```python
from build123d import *

# Parameters (mm, degrees)
BOSS_EXTRUDE1_START     = -2.5
SKETCH1_W               = 70
SKETCH1_H               = 39.95
BOSS_EXTRUDE1_DEPTH     = 2.5
SKETCH2_W               = 60
SKETCH2_H               = 2.6
BOSS_EXTRUDE2_DEPTH     = 13.5
SKETCH3_W               = 60
SKETCH3_H               = 2.6
BOSS_EXTRUDE3_DEPTH     = 13.5
SKETCH4_R               = 2.75
BOSS_EXTRUDE4_DEPTH     = 13.5
BOSS_EXTRUDE5_START     = -19
SKETCH5_R               = 5
BOSS_EXTRUDE5_DEPTH     = 16.5
SKETCH6_R               = 3
BOSS_EXTRUDE6_DEPTH     = 22.6
CUT_EXTRUDE1_START      = 14.6
SKETCH7_R               = 0.9
CUT_EXTRUDE1_DEPTH      = 8.1
CUT_EXTRUDE2_DEPTH      = 47.965525921
CUT_EXTRUDE2_DEPTH_BACK = 47.965525921
SKETCH8_W               = 22.8
SKETCH8_H               = 11.9
CUT_EXTRUDE3_DEPTH      = 47.965525921
CUT_EXTRUDE3_DEPTH_BACK = 47.965525921
SKETCH9_R               = 0.9
CUT_EXTRUDE4_DEPTH      = 47.965525921
CUT_EXTRUDE4_DEPTH_BACK = 47.965525921
SKETCH10_R              = 0.9
CUT_EXTRUDE5_DEPTH      = 47.965525921
CUT_EXTRUDE5_DEPTH_BACK = 47.965525921
SKETCH11_R              = 1.725
CUT_EXTRUDE6_START      = -4.2
CUT_EXTRUDE6_DEPTH      = 4.2


with BuildPart() as part:
    # Sketch1 → Boss-Extrude1 (new body)
    with BuildSketch(Plane.XY.offset(BOSS_EXTRUDE1_START)):
        Rectangle(SKETCH1_W, SKETCH1_H)
    extrude(amount=BOSS_EXTRUDE1_DEPTH)

    # Sketch2 → Boss-Extrude2 (add)
    with BuildSketch(Plane.XY):
        with Locations((-5, 16.975)):
            Rectangle(SKETCH2_W, SKETCH2_H)
    extrude(amount=BOSS_EXTRUDE2_DEPTH)

    # Sketch3 → Boss-Extrude3 (add)
    with BuildSketch(Plane.XY):
        with Locations((5, -16.975)):
            Rectangle(SKETCH3_W, SKETCH3_H)
    extrude(amount=BOSS_EXTRUDE3_DEPTH)

    # Sketch4 → Boss-Extrude4 (add)
    with BuildSketch(Plane.XY):
        with Locations((-8, 16.975)):
            Circle(SKETCH4_R)
        with Locations((8, -16.975)):
            Circle(SKETCH4_R)
    extrude(amount=BOSS_EXTRUDE4_DEPTH)

    # Sketch5 → Boss-Extrude5 (add)
    with BuildSketch(Plane.XY.offset(BOSS_EXTRUDE5_START)):
        with Locations(Location((-31, 6, 0), (0, 0, 143.130102354))):
            Circle(SKETCH5_R)
        with Locations(Location((-31, -6, 0), (0, 0, 143.130102354))):
            Circle(SKETCH5_R)
    extrude(amount=BOSS_EXTRUDE5_DEPTH)

    # Sketch6 → Boss-Extrude6 (add)
    with BuildSketch(Plane.XY):
        with Locations((30, 0)):
            Circle(SKETCH6_R)
        with Locations((-30, 0)):
            Circle(SKETCH6_R)
    extrude(amount=BOSS_EXTRUDE6_DEPTH)

    # Sketch7 → Cut-Extrude1 (cut)
    with BuildSketch(Plane.XY.offset(CUT_EXTRUDE1_START)):
        with Locations((30, 0)):
            Circle(SKETCH7_R)
        with Locations((-30, 0)):
            Circle(SKETCH7_R)
    extrude(amount=CUT_EXTRUDE1_DEPTH, mode=Mode.SUBTRACT)

    # Sketch8 → Cut-Extrude2 (cut, two sides: drawn at the far end of the back side and taken through both)
    with BuildSketch(Plane.XY.offset(-CUT_EXTRUDE2_DEPTH_BACK)):
        with Locations((5.8, 0)):
            Rectangle(SKETCH8_W, SKETCH8_H)
    extrude(amount=CUT_EXTRUDE2_DEPTH + CUT_EXTRUDE2_DEPTH_BACK, mode=Mode.SUBTRACT)

    # Sketch9 → Cut-Extrude3 (cut, two sides: drawn at the far end of the back side and taken through both)
    with BuildSketch(Plane.XY.offset(-CUT_EXTRUDE3_DEPTH_BACK)):
        with Locations((-7.95, 0)):
            Circle(SKETCH9_R)
        with Locations((19.55, 0)):
            Circle(SKETCH9_R)
    extrude(amount=CUT_EXTRUDE3_DEPTH + CUT_EXTRUDE3_DEPTH_BACK, mode=Mode.SUBTRACT)

    # Sketch10 → Cut-Extrude4 (cut, two sides: drawn at the far end of the back side and taken through both)
    with BuildSketch(Plane.XY.offset(-CUT_EXTRUDE4_DEPTH_BACK)):
        with Locations((-8, 16.975)):
            Circle(SKETCH10_R)
        with Locations((8, -16.975)):
            Circle(SKETCH10_R)
    extrude(amount=CUT_EXTRUDE4_DEPTH + CUT_EXTRUDE4_DEPTH_BACK, mode=Mode.SUBTRACT)

    # Sketch11 → Cut-Extrude5 (cut, two sides: drawn at the far end of the back side and taken through both)
    with BuildSketch(Plane.XY.offset(-CUT_EXTRUDE5_DEPTH_BACK)):
        with Locations((-31, 6)):
            Circle(SKETCH11_R)
        with Locations((-31, -6)):
            Circle(SKETCH11_R)
    extrude(amount=CUT_EXTRUDE5_DEPTH + CUT_EXTRUDE5_DEPTH_BACK, mode=Mode.SUBTRACT)

    # Sketch12 → Cut-Extrude6 (cut)
    with BuildSketch(Plane.XY.offset(CUT_EXTRUDE6_START)):
        Polygon((-28.2, 7.616580754), (-31, 9.233161507), (-33.8, 7.616580754), (-33.8, 4.383419246), (-31, 2.766838493), (-28.2, 4.383419246), align=None)
        Polygon((-28.2, -4.383419246), (-31, -2.766838493), (-33.8, -4.383419246), (-33.8, -7.616580754), (-31, -9.233161507), (-28.2, -7.616580754), align=None)
    extrude(amount=CUT_EXTRUDE6_DEPTH, mode=Mode.SUBTRACT)


solid = part.part
```
For this review, take the finished solid that the model builds, in its own axes (mm). A direction names the side the tool comes from. Coordinates: 2 decimals unless noted, no trailing zeros. Loops run counter-clockwise (first coordinate to the right, second up) from the corner with the lowest first, then second, coordinate; pieces in that order, holes last. Notation, with made-up numbers: (69, 7.25) -> (120, 7.25) arc R21 ccw to (120, 30.25) -> close; hole circle Ø4 at (-13.75, 39). An arc over 180 degrees is marked (long way). Return JSON: item names as keys, results as strings. Group by question number.
(1) Consider section B-B, the plane x = 13.5. Give the boundary of the cut face in (y, z) (3 decimals), plus the area to 3 significant figures.
(2) Tool access review of faces 4 (the cylindrical face through (8.042, -14.225, 6.656)), 5 (the flat face through (-25, -17, 7)), 6 (the flat face through (-35, 5.8, -0.5)): name each direction out of +Z, -Z, +X, -X, +Y, -Y from which nothing blocks a thin tool from reaching the whole face with its end or side.
(3) Consider section C-C, the plane y = 0. Count the separate pieces of the cut face and the enclosed holes in it, plus the area to 3 significant figures.
(4) For pin 1 Ø0.8 at (y, z) = (2, -1) entering from -X; pin 2 Ø10 at (x, y) = (16.5, 15) entering from +Z; pin 3 Ø10 at (x, y) = (24.5, -13) entering from -Z, all flat-tipped, find the tip position at first contact; note any pin that passes through.
(5) Consider section D-D, the plane x = 30. Give the boundary of the cut face in (y, z) (3 decimals).
(6) Consider section A-A, the plane z = -14. Give the boundary of the cut face in (x, y) (3 decimals).
(7) To check wall thickness, follow L1, parallel to Y at x = -31, z = -15.25 (3 decimals); L2, parallel to X at y = 0, z = -1.25; L3, parallel to X at y = 6, z = -13 (3 decimals). State the ranges of each line that lie inside material, in increasing order.
(8) Mouldability with a two-part tool opening along Y and no side actions: class faces 1 (the flat face through (25, 17, 7)), 2 (the cylindrical face through (27, 0, 11)), 3 (the cylindrical face through (-7.958, 19.725, 6.656)) as pulls with the +Y half, pulls with the -Y half, needs draft (parallel to the pull), parting line crosses it, or undercut.
Results below:
{
 "1": {"outline": "(-19.975, -2.5) -> (-5.95, -2.5) -> (-5.95, 0) -> (-15.675, 0) -> (-15.675, 13.5) -> (-18.275, 13.5) -> (-18.275, 0) -> (-19.975, 0) -> close; (5.95, -2.5) -> (19.975, -2.5) -> (19.975, 0) -> (18.275, 0) -> (18.275, 13.5) -> (15.675, 13.5) -> (15.675, 0) -> (5.95, 0) -> close", "area": "140 mm2"},
 "2": {"face 4": "+Z", "face 5": "+Z, -X, -Y", "face 6": "+Z, -X, +Y, -Y"},
 "3": {"separate pieces": "4", "enclosed holes": "0", "area": "351 mm2"},
 "4": {"pin 1": "stops at x = -35", "pin 2": "stops at z = 13.5", "pin 3": "stops at z = -2.5"},
 "5": {"outline": "(-19.975, -2.5) -> (19.975, -2.5) -> (19.975, 0) -> (3, 0) -> (3, 22.6) -> (0.9, 22.6) -> (0.9, 14.6) -> (-0.9, 14.6) -> (-0.9, 22.6) -> (-3, 22.6) -> (-3, 0) -> (-15.675, 0) -> (-15.675, 13.5) -> (-18.275, 13.5) -> (-18.275, 0) -> (-19.975, 0) -> close"},
 "6": {"outline": "circle Ø10 at (-31, -6); circle Ø10 at (-31, 6); hole circle Ø3.45 at (-31, -6); hole circle Ø3.45 at (-31, 6)"},
 "7": {"L1": "y = -11 to -7.725, -4.275 to -1, 1 to 4.275, 7.725 to 11", "L2": "x = -35 to -8.85, -7.05 to -5.6, 17.2 to 18.65, 20.45 to 35", "L3": "x = -36 to -32.725, -29.275 to -26"},
 "8": {"face 1": "needs draft", "face 2": "undercut", "face 3": "pulls with the +Y half"}
}
